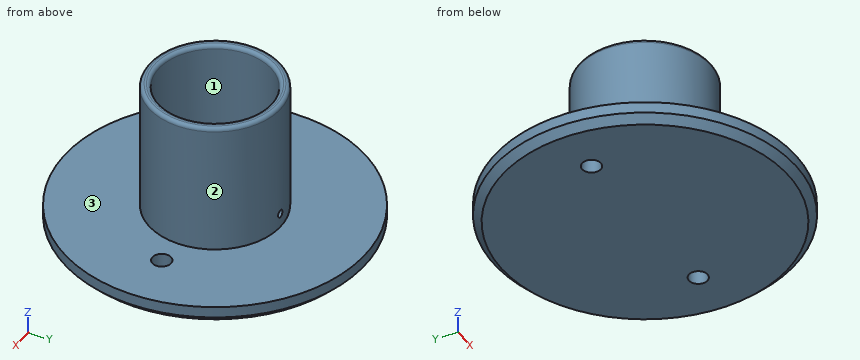
from build123d import *

# Parameters (mm, degrees)
F0_R     = 25.4
F0_R_2   = 1.5785092345
F1_DEPTH = 3.175
F2_DEPTH = 25.4
F3_R     = 0.635
F4_DEPTH = 25.4
F5_SIZE  = 1.27
F6_R     = 0.635


with BuildPart() as f1:
    # F0 (on Top) → F1 (new body)
    with BuildSketch(Plane.XY):
        Circle(F0_R)
        with Locations((-15.9070281119, 0)):
            Circle(F0_R_2, mode=Mode.SUBTRACT)
        with BuildLine():
            ThreePointArc((-11.1093761475, 0), (0, 11.1093761475), (11.1093761475, 0))
            ThreePointArc((11.1093761475, 0), (0, -11.1093761475), (-11.1093761475, 0))
        make_face(mode=Mode.SUBTRACT)
        with BuildLine():
            ThreePointArc((17.4326761663, 0), (15.8555379837, -1.5771381826), (14.2783998011, 0))
            ThreePointArc((14.2783998011, 0), (15.8555379837, 1.5771381826), (17.4326761663, 0))
        make_face(mode=Mode.SUBTRACT)
        with BuildLine():
            Line((0, 0), (9.5014704661, 0))
            ThreePointArc((9.5014704661, 0), (0, 9.5014704661), (-9.5014704661, 0))
            Line((-9.5014704661, 0), (0, 0))
        make_face()
        with BuildLine():
            ThreePointArc((-9.5014704661, 0), (0, -9.5014704661), (9.5014704661, 0))
            Line((9.5014704661, 0), (0, 0))
            Line((0, 0), (-9.5014704661, 0))
        make_face()
        with BuildLine():
            ThreePointArc((-9.5014704661, 0), (0, 9.5014704661), (9.5014704661, 0))
            Line((9.5014704661, 0), (11.1093761475, 0))
            ThreePointArc((11.1093761475, 0), (0, 11.1093761475), (-11.1093761475, 0))
            Line((-11.1093761475, 0), (-9.5014704661, 0))
        make_face()
        with BuildLine():
            Line((11.1093761475, 0), (9.5014704661, 0))
            ThreePointArc((9.5014704661, 0), (0, -9.5014704661), (-9.5014704661, 0))
            Line((-9.5014704661, 0), (-11.1093761475, 0))
            ThreePointArc((-11.1093761475, 0), (0, -11.1093761475), (11.1093761475, 0))
        make_face()
    extrude(amount=F1_DEPTH)

    # F0 (on Top) → F2 (join)
    with BuildSketch(Plane.XY):
        with BuildLine():
            Line((11.1093761475, 0), (9.5014704661, 0))
            ThreePointArc((9.5014704661, 0), (0, -9.5014704661), (-9.5014704661, 0))
            Line((-9.5014704661, 0), (-11.1093761475, 0))
            ThreePointArc((-11.1093761475, 0), (0, -11.1093761475), (11.1093761475, 0))
        make_face()
        with BuildLine():
            ThreePointArc((-9.5014704661, 0), (0, 9.5014704661), (9.5014704661, 0))
            Line((9.5014704661, 0), (11.1093761475, 0))
            ThreePointArc((11.1093761475, 0), (0, 11.1093761475), (-11.1093761475, 0))
            Line((-11.1093761475, 0), (-9.5014704661, 0))
        make_face()
    extrude(amount=F2_DEPTH)

    # F3 (on Front) → F4 (cut)
    with BuildSketch(Plane.XZ):
        with Locations((0, 5.5941580795)):
            Circle(F3_R)
    extrude(amount=-F4_DEPTH, mode=Mode.SUBTRACT)

    # F5
    f5_edges = [f1.edges().sort_by_distance(p)[0] for p in [
        (-25.4, 0, 0),
    ]]
    chamfer(f5_edges, length=F5_SIZE)

    # F6
    f6_edges = [f1.edges().sort_by_distance(p)[0] for p in [
        (-11.109376, 0, 25.4),
        (9.50147, 0, 25.4),
    ]]
    fillet(f6_edges, radius=F6_R)


solid = f1.part
Verification items for the finished model (mm, model axes). Face numbers are marked on the shaded views. Coordinates: 2 decimals unless noted, no trailing zeros. Write each loop counter-clockwise with the first axis right and the second up, starting at its lowest first coordinate (ties: lowest second). Pieces come first, ordered by that corner, then holes. Notation, with made-up numbers: (-32, -34) -> (-18, -34) arc R18 cw to (-18, -20) -> close; hole circle Ø2 at (23, 24). An arc over 180 degrees is marked (long way). One line per item, written item: value. Start each with the question number.
Q1. Thickness scan on L1, parallel to Y at x = 0, z = 10.5; L2, parallel to Z at x = -6.5, y = -10 (3 decimals); L3, parallel to X at y = 7, z = 7.25. Record the ranges inside material, lowest first. Write a range as from..to.
Q2. Mould release check, pull along X, two halves, no side actions. Record for the marked faces 1, 2 and 3: pulls with the +X half, pulls with the -X half, needs draft (parallel to the pull), parting line crosses it, or undercut.
Q3. Cross-section at A-A on y = 0. Enter the section's corners in (x, z) (3 decimals).
Q4. Go/stop test with flat-tipped pins: P1, Ø8, axis at x = -14.5, y = 16, coming from the +Z side (3 decimals); P2, Ø3, axis at x = 8.5, z = 9.5, coming from the +Y side; P3, Ø12, axis at y = -10.5, z = 13, coming from the +X side; P4, Ø12, axis at x = -19, y = -14, coming from the -Z side. Record where each tip stops, or that it passes through.
Q5. Cross-section at C-C on z = 20.25. Enter the section's corners in (x, y).
Q6. Cross-section at B-B on x = 0. Enter the section's corners in (y, z) (3 decimals), and give its area (3 significant figures).
Checked values:
1. L1: y = -11.11..-9.5, 9.5..11.11
1. L2: z = 0..3.175
1. L3: x = -8.63..-6.42, 6.42..8.63
2. face 1: undercut
2. face 2: parting line crosses it
2. face 3: needs draft
3. outline: (-25.4, 1.27) -> (-24.13, 0) -> (-17.486, 0) -> (-17.486, 3.175) -> (-25.4, 3.175) -> close; (-14.329, 0) -> (14.278, 0) -> (14.278, 3.175) -> (11.109, 3.175) -> (11.109, 24.765) arc R0.635 ccw to (10.474, 25.4) -> (10.136, 25.4) arc R0.635 ccw to (9.501, 24.765) -> (9.501, 3.175) -> (-9.501, 3.175) -> (-9.501, 24.765) arc R0.635 ccw to (-10.136, 25.4) -> (-10.474, 25.4) arc R0.635 ccw to (-11.109, 24.765) -> (-11.109, 3.175) -> (-14.329, 3.175) -> close; (17.433, 0) -> (24.13, 0) -> (25.4, 1.27) -> (25.4, 3.175) -> (17.433, 3.175) -> close
4. P1: stops at z = 3.175
4. P2: stops at y = 8.63
4. P3: stops at x = 10.16
4. P4: stops at z = 0
5. outline: circle Ø22.22 at (0, 0); hole circle Ø19 at (0, 0)
6. outline: (-25.4, 1.27) -> (-24.13, 0) -> (24.13, 0) -> (25.4, 1.27) -> (25.4, 3.175) -> (11.109, 3.175) -> (11.109, 4.959) -> (9.501, 4.959) -> (9.501, 3.175) -> (-9.501, 3.175) -> (-9.501, 24.765) arc R0.635 ccw to (-10.136, 25.4) -> (-10.474, 25.4) arc R0.635 ccw to (-11.109, 24.765) -> (-11.109, 3.175) -> (-25.4, 3.175) -> close; (9.501, 6.229) -> (11.109, 6.229) -> (11.109, 24.765) arc R0.635 ccw to (10.474, 25.4) -> (10.136, 25.4) arc R0.635 ccw to (9.501, 24.765) -> close
6. area: 229 mm²
